The listing builds one solid part. Answer for the finished solid, in the listing's coordinates (mm). A direction names the side the tool comes from. Coordinates: 2 decimals unless noted, no trailing zeros. Write each loop counter-clockwise with the first axis right and the second up, starting at its lowest first coordinate (ties: lowest second). Pieces come first, ordered by that corner, then holes.
from build123d import *

# Parameters (mm, degrees)
SKETCH1_R           = 127
SKETCH1_R_2         = 63.5
BOSS_EXTRUDE1_DEPTH = 5.334
SKETCH14_R          = 3.175
BOLTHOLES_DEPTH     = 180.684310823
SKETCH15_W          = 2.4638
SKETCH15_H          = 19.05
SKETCH15_W_2        = 5.334
MOTORMOUNTS_DEPTH   = 180.684310823


with BuildPart() as part:
    # Sketch1 → Boss-Extrude1 (new body)
    # profile 1 of 3: a face of its own
    with BuildSketch(Plane.XY):
        Circle(SKETCH1_R)
        Circle(SKETCH1_R_2, mode=Mode.SUBTRACT)
    # profile 2 of 3: a face of its own
    with BuildSketch(Plane.XY):
        with BuildLine():
            Line((-40.299999918, -49.073006904), (-40.299999918, 49.073006904))
            ThreePointArc((-40.299999918, 49.073006904), (-63.5, 0), (-40.299999918, -49.073006904))
        make_face()
    # profile 3 of 3: a face of its own
    with BuildSketch(Plane.XY):
        with BuildLine():
            ThreePointArc((63.5, 0), (57.407752067, 27.140375874), (40.299999918, 49.073006904))
            Line((40.299999918, 49.073006904), (40.299999918, -49.073006904))
            ThreePointArc((40.299999918, -49.073006904), (57.407752067, -27.140375874), (63.5, 0))
        make_face()
    extrude(amount=BOSS_EXTRUDE1_DEPTH)

    # Sketch14 → BoltHoles (cut, through all)
    with BuildSketch(Plane.XY.offset(5.334)):
        with Locations((-76.2, -78.74)):
            Circle(SKETCH14_R)
        with Locations((-50.8, 78.74)):
            Circle(SKETCH14_R)
        with Locations(Location((76.2, -78.74, 0), (0, 0, 180))):
            Circle(SKETCH14_R)
        with Locations(Location((50.8, 78.74, 0), (0, 0, 180))):
            Circle(SKETCH14_R)
    extrude(amount=-BOLTHOLES_DEPTH, mode=Mode.SUBTRACT)

    # Sketch15 → MotorMounts (cut, through all)
    with BuildSketch(Plane.XY.offset(5.334)):
        with Locations((-100.3681, -41.275)):
            Rectangle(SKETCH15_W, SKETCH15_H)
        with Locations((-100.3681, 0)):
            Rectangle(SKETCH15_W, SKETCH15_H)
        with Locations((-78.469199932, -41.275)):
            Rectangle(SKETCH15_W_2, SKETCH15_H)
        with Locations((-42.966999918, -41.275)):
            Rectangle(SKETCH15_W_2, SKETCH15_H)
        with Locations((-78.469199932, 0)):
            Rectangle(SKETCH15_W_2, SKETCH15_H)
        with Locations((42.966999918, 0)):
            Rectangle(SKETCH15_W_2, SKETCH15_H)
        with Locations((42.966999918, -41.275)):
            Rectangle(SKETCH15_W_2, SKETCH15_H)
        with Locations((78.469199932, 0)):
            Rectangle(SKETCH15_W_2, SKETCH15_H)
        with Locations((100.3681, 0)):
            Rectangle(SKETCH15_W, SKETCH15_H)
        with Locations((-42.966999918, 0)):
            Rectangle(SKETCH15_W_2, SKETCH15_H)
        with Locations((78.469199932, -41.275)):
            Rectangle(SKETCH15_W_2, SKETCH15_H)
        with Locations((100.3681, -41.275)):
            Rectangle(SKETCH15_W, SKETCH15_H)
    extrude(amount=-MOTORMOUNTS_DEPTH, mode=Mode.SUBTRACT)


solid = part.part
1. For a pull along Y with two mould halves and no side action, classify faces 3 (the cylindrical face through (-27.53, -123.98, 2.63)), 4 (the flat face through (55, 2, 5.334)), 5 (the cylindrical face through (74.493, -81.417, 2.704)) as pulls with the +Y half, pulls with the -Y half, needs draft (parallel to the pull), parting line crosses it, or undercut.
Results found:
face 3: parting line crosses it
face 4: needs draft
face 5: undercut
2. A tool of negligible diameter and unlimited length cuts with its end or side. For faces 1 (the flat face through (55, 2, 0)), 2 (the cylindrical face through (0.611, 63.497, 2.63)), from which of +Z, -Z, +X, -X, +Y, -Y can it reach the whole face along a straight path? Write none if from no direction.
Results found:
face 1: -Z, +X, -X, +Y, -Y
face 2: +Z, -Z
3. Find the intervals of material crossed by L1, parallel to Y at x = -76.2, z = 1.2 (3 decimals); L2, parallel to X at y = -3, z = 0.4; L3, parallel to X at y = -81, z = 1.05, in increasing order.
Results found:
L1: y = -101.6 to -81.915, -75.565 to -50.8, -31.75 to -9.525, 9.525 to 101.6
L2: x = -126.96 to -101.6, -99.14 to -81.14, -75.8 to -45.63, 45.63 to 75.8, 81.14 to 99.14, 101.6 to 126.96
L3: x = -97.82 to -78.43, -73.97 to 73.97, 78.43 to 97.82
4. Section C-C on y = 78.74 is taken. Give the vertices of the cut face in (x, z) (3 decimals).
Results found:
outline: (-99.644, 0) - (-53.975, 0) - (-53.975, 5.334) - (-99.644, 5.334) - close; (-47.625, 0) - (47.625, 0) - (47.625, 5.334) - (-47.625, 5.334) - close; (53.975, 0) - (99.644, 0) - (99.644, 5.334) - (53.975, 5.334) - close
5. Section A-A on x = 0 is taken. Give the vertices of the cut face in (y, z), then the cut area to 3 significant figures.
Results found:
outline: (-127, 0) - (-63.5, 0) - (-63.5, 5.33) - (-127, 5.33) - close; (63.5, 0) - (127, 0) - (127, 5.33) - (63.5, 5.33) - close
area: 677 mm2
6. Section D-D on z = 3.5 is taken. State how many separate pieces and enclosed holes the cut face has, then the cut area to 3 significant figures.
Results found:
separate pieces: 1
enclosed holes: 13
area: 40,000 mm2
7. Flat-ended cylindrical pins translate along their axes: P1, Ø1.6, axis at y = 4.5, z = 2.5, coming from the +X side; P2, Ø1.6, axis at x = 79, z = 4, coming from the +Y side; P3, Ø2, axis at x = 100.5, z = 3.5, coming from the +Y side. Find the tip coordinate at first contact, or state that the pin passes through.
Results found:
P1: stops at x = 126.95
P2: stops at y = 100.07
P3: stops at y = 78.92
8. Section B-B on y = 24 is taken. Give the vertices of the cut face in (x, z).
Results found:
outline: (-124.71, 0) - (-40.3, 0) - (-40.3, 5.33) - (-124.71, 5.33) - close; (40.3, 0) - (124.71, 0) - (124.71, 5.33) - (40.3, 5.33) - close
